Check sheet for the modelled part. Datum: model origin and axes. Units: mm. A direction names the side the tool comes from. Give positions to 0.01 mm unless a question says otherwise; leave off trailing zeros. Order: outer loops, then holes, each group sorted by start corner. A loop starts at its lowest first (then second) coordinate and runs counter-clockwise, first axis right, second up. Notation, with made-up numbers: (47, 69.25) -> (63, 69.25) arc R9 ccw to (63, 85.25) -> close; hole circle Ø8 at (17.25, 48). An arc over 180 degrees is marked (long way). Answer in a Markdown table with one row per item. Add a question column.
(1) Thickness scan on L1, parallel to Y at x = 0, z = -20; L2, parallel to X at y = 3.5, z = -10.5; L3, parallel to X at y = -8.5, z = -39. Record the ranges inside material, lowest first. Write a range as [from, to].
(2) Cross-section at A-A (x = -12). Record the cut outline in (y, z), then the cut area to 3 significant figures.
(3) Go/stop test with flat-tipped pins: pin 1 (0.8 mm diameter, centred on y = -14, z = -13.5, fed in from +X); pin 2 (3.5 mm diameter, centred on x = -2.5, z = -22.5, fed in from -Y). Record where each tip stops, or that it passes through.
(4) Release check for a two-part mould opening along Y. For faces 1 (the face through (-12.269, 13.624, -24.65)), 2 (the face through (4, -14, -25)), 3 (the face through (0, 15, -25)) record: released by +Y, released by -Y, zero draft, split by the parting line, or undercut.
(5) Cross-section at C-C (z = -31). State how many separate pieces and enclosed holes the cut face has, then the cut area to 3 significant figures.
(6) Cross-section at B-B (y = 9). Record the cut outline in (x, z).
(7) Set-up check for faces 4 (the face through (-6, -13, -25)), 5 (the face through (-14.4, 14.43, -24.65)), 6 (the face through (-3.905, -0.867, -2.028)): record each of +Z, -Z, +X, -X, +Y, -Y from which the full face is reachable in a straight line by a thin tool's end or side.
```python
from build123d import *

# Parameters (mm, degrees)
SKETCH1_R           = 2.1
SKETCH1_R_2         = 3.4
BOSS_EXTRUDE1_DEPTH = 50
SKETCH3_W           = 2
SKETCH3_H           = 9.175206629
SKETCH3_W_2         = 11.07645362
SKETCH3_H_2         = 2
SKETCH3_H_3         = 11.915453224
BOSS_EXTRUDE2_DEPTH = 50
SKETCH4_W           = 3
SKETCH4_H           = 21.746320034
CUT_EXTRUDE1_DEPTH  = 51


with BuildPart() as part:
    # Sketch1 → Boss-Extrude1 (new body)
    with BuildSketch(Plane.XY):
        with BuildLine():
            Line((-15, 13), (-15, 4.3))
            ThreePointArc((-15, 4.3), (-14.912132034, 4.087867966), (-14.7, 4))
            Line((-14.7, 4), (-13, 4))
            Line((-13, 4), (-13, 8.25))
            Line((-13, 8.25), (-9.6642, 8.25))
            Line((-9.6642, 8.25), (-6, 4.5858))
            Line((-6, 4.5858), (-6, 0.519615242))
            Line((-6, 0.519615242), (-5.7, 0))
            Line((-5.7, 0), (-6, -0.519615242))
            Line((-6, -0.519615242), (-6, -4.5858))
            Line((-6, -4.5858), (-9.6642, -8.25))
            Line((-9.6642, -8.25), (-13, -8.25))
            Line((-13, -8.25), (-13, -4))
            Line((-13, -4), (-14.7, -4))
            ThreePointArc((-14.7, -4), (-14.912132034, -4.087867966), (-15, -4.3))
            Line((-15, -4.3), (-15, -13))
            ThreePointArc((-15, -13), (-14.414213562, -14.414213562), (-13, -15))
            Line((-13, -15), (-4.3, -15))
            ThreePointArc((-4.3, -15), (-4.087867966, -14.912132034), (-4, -14.7))
            Line((-4, -14.7), (-4, -13))
            Line((-4, -13), (-8.25, -13))
            Line((-8.25, -13), (-8.25, -9.6642))
            Line((-8.25, -9.6642), (-4.5858, -6))
            Line((-4.5858, -6), (-0.519615242, -6))
            Line((-0.519615242, -6), (0, -5.7))
            Line((0, -5.7), (0.519615242, -6))
            Line((0.519615242, -6), (4.5858, -6))
            Line((4.5858, -6), (8.25, -9.6642))
            Line((8.25, -9.6642), (8.25, -13))
            Line((8.25, -13), (4, -13))
            Line((4, -13), (4, -14.7))
            ThreePointArc((4, -14.7), (4.087867966, -14.912132034), (4.3, -15))
            Line((4.3, -15), (13, -15))
            ThreePointArc((13, -15), (14.414213562, -14.414213562), (15, -13))
            Line((15, -13), (15, -4.3))
            ThreePointArc((15, -4.3), (14.912132034, -4.087867966), (14.7, -4))
            Line((14.7, -4), (13, -4))
            Line((13, -4), (13, -8.25))
            Line((13, -8.25), (9.6642, -8.25))
            Line((9.6642, -8.25), (6, -4.5858))
            Line((6, -4.5858), (6, -0.519615242))
            Line((6, -0.519615242), (5.7, 0))
            Line((5.7, 0), (6, 0.519615242))
            Line((6, 0.519615242), (6, 4.5858))
            Line((6, 4.5858), (9.6642, 8.25))
            Line((9.6642, 8.25), (13, 8.25))
            Line((13, 8.25), (13, 4))
            Line((13, 4), (14.7, 4))
            ThreePointArc((14.7, 4), (14.912132034, 4.087867966), (15, 4.3))
            Line((15, 4.3), (15, 13))
            ThreePointArc((15, 13), (14.414213562, 14.414213562), (13, 15))
            Line((13, 15), (4.3, 15))
            ThreePointArc((4.3, 15), (4.087867966, 14.912132034), (4, 14.7))
            Line((4, 14.7), (4, 13))
            Line((4, 13), (8.25, 13))
            Line((8.25, 13), (8.25, 9.6642))
            Line((8.25, 9.6642), (4.5858, 6))
            Line((4.5858, 6), (0.519615242, 6))
            Line((0.519615242, 6), (0, 5.7))
            Line((0, 5.7), (-0.519615242, 6))
            Line((-0.519615242, 6), (-4.5858, 6))
            Line((-4.5858, 6), (-8.25, 9.6642))
            Line((-8.25, 9.6642), (-8.25, 13))
            Line((-8.25, 13), (-4, 13))
            Line((-4, 13), (-4, 14.7))
            ThreePointArc((-4, 14.7), (-4.087867966, 14.912132034), (-4.3, 15))
            Line((-4.3, 15), (-13, 15))
            ThreePointArc((-13, 15), (-14.414213562, 14.414213562), (-15, 13))
        make_face()
        with Locations((11.625, -11.625)):
            Circle(SKETCH1_R, mode=Mode.SUBTRACT)
        with Locations((11.625, 11.625)):
            Circle(SKETCH1_R, mode=Mode.SUBTRACT)
        Circle(SKETCH1_R_2, mode=Mode.SUBTRACT)
        with Locations((-11.625, -11.625)):
            Circle(SKETCH1_R, mode=Mode.SUBTRACT)
        with Locations((-11.625, 11.625)):
            Circle(SKETCH1_R, mode=Mode.SUBTRACT)
    extrude(amount=-BOSS_EXTRUDE1_DEPTH)

    # Sketch2 → Cut-Revolve1 (revolve, cut)
    with BuildSketch(Plane(origin=(0, 0, 0), x_dir=(-1, 0, 0), z_dir=(0, 1, 0))):
        Polygon((0, -28.31882362), (-3.3235, -26.4), (-3.3235, -0.6765), (-4, 0), (0, 0), align=None)
    revolve(axis=Axis((0, 0, 0), (0, 0, -1)), mode=Mode.SUBTRACT)

    # Sketch3 → Boss-Extrude2 (add)
    with BuildSketch(Plane.XY):
        with Locations((-14, -0.287603314)):
            Rectangle(SKETCH3_W, SKETCH3_H)
        with Locations((-0.643781897, 14)):
            Rectangle(SKETCH3_W_2, SKETCH3_H_2)
        with Locations((14, -0.392977161)):
            Rectangle(SKETCH3_W, SKETCH3_H_3)
    extrude(amount=-BOSS_EXTRUDE2_DEPTH)

    # Sketch4 → Cut-Extrude1 (cut, through all)
    with BuildSketch(Plane.XY):
        with Locations((11.1642, 0)):
            Rectangle(SKETCH4_W, SKETCH4_H)
        with Locations((-11.1642, 0)):
            Rectangle(SKETCH4_W, SKETCH4_H)
    extrude(amount=-CUT_EXTRUDE1_DEPTH, mode=Mode.SUBTRACT)

    # Sketch5 → Cut-Revolve5 (revolve, cut)
    with BuildSketch(Plane(origin=(0, 0, 0), x_dir=(0, 0, -1), z_dir=(1, 0, 0))):
        Polygon((0, 0), (0, 4), (4, 4), (6.309401077, 0), align=None)
    revolve(axis=Axis((0, 0, 0), (0, 0, -1)), mode=Mode.SUBTRACT)


solid = part.part
```
Answer below:
| question | item | result |
|---|---|---|
| 1 | L1 | y = [-5.7, -3.4], [3.4, 5.7], [13, 15] |
| 1 | L2 | x = [-15, -13], [-6, 6], [13, 15] |
| 1 | L3 | x = [-15, -12.66], [-9.66, -7.09], [7.09, 9.66], [12.66, 15] |
| 2 | outline | (-15, -50) -> (-13.69, -50) -> (-13.69, 0) -> (-15, 0) -> close; (13.69, -50) -> (15, -50) -> (15, 0) -> (13.69, 0) -> close |
| 2 | area | 131 mm² |
| 3 | pin 1 | stops at x = 14.91 |
| 3 | pin 2 | stops at y = -15 |
| 4 | face 1 | undercut |
| 4 | face 2 | zero draft |
| 4 | face 3 | released by +Y |
| 5 | separate pieces | 1 |
| 5 | enclosed holes | 4 |
| 5 | area | 361 mm² |
| 6 | outline | (-15, -50) -> (-12.66, -50) -> (-12.66, 0) -> (-15, 0) -> close; (-9.66, -50) -> (-7.59, -50) -> (-7.59, 0) -> (-9.66, 0) -> close; (7.59, -50) -> (9.66, -50) -> (9.66, 0) -> (7.59, 0) -> close; (12.66, -50) -> (15, -50) -> (15, 0) -> (12.66, 0) -> close |
| 7 | face 4 | +Z, -Z |
| 7 | face 5 | +Z, -Z, -X, +Y |
| 7 | face 6 | +Z |
